Here's the drawing with two shaded views (mm, measured from the low corner). I have some questions. A direction names the side the tool comes from. Round coordinates to 2 decimals unless told otherwise and drop trailing zeros. Order: outer loops, then holes, each group sorted by start corner. A loop starts at its lowest first (then second) coordinate and runs counter-clockwise, first axis right, second up. Notation, with made-up numbers: (-24.5, -10) - (3.5, -10) arc R18 cw to (3.5, 6) - close; hole circle Ø7 at (0, 66). An arc over 180 degrees is marked (long way). One line per item, written item: value.
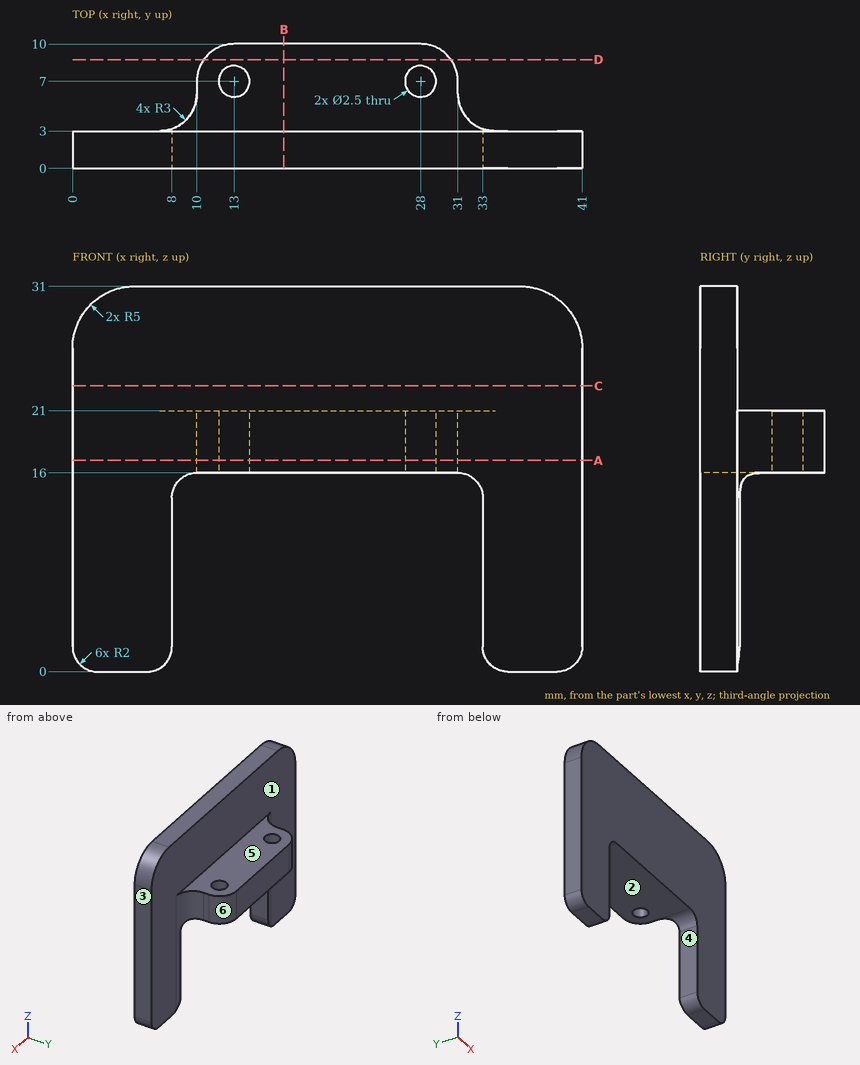
Q1. If we section it at C-C, the plane z = 23: Please give me the cut outline in (x, y), then the cut area to 3 significant figures.
Results list:
outline: (0, 0) - (41, 0) - (41, 3) - (0, 3) - close
area: 123 mm²
Q2. Will these pins go through, and if not, where does the flat tip stop? pin 1 (5.5 mm diameter, centred on x = 26.5, y = 5.5, fed in from +Z); pin 2 (1 mm diameter, centred on x = 29, z = 27.5, fed in from +Y); pin 3 (3 mm diameter, centred on x = 18.5, y = 6.5, fed in from -Z); pin 4 (0.8 mm diameter, centred on y = 6.5, z = 19, fed in from -X).
Results list:
pin 1: z = 31
pin 2: y = 3
pin 3: z = 16
pin 4: x = 10
Q3. If we section it at A-A, the plane z = 17: Please give me the cut outline in (x, y), then the cut area to 3 significant figures.
Results list:
outline: (0, 0) - (41, 0) - (41, 3) - (34, 3) arc R3 cw to (31, 6) - (31, 7) arc R3 ccw to (28, 10) - (13, 10) arc R3 ccw to (10, 7) - (10, 6) arc R3 cw to (7, 3) - (0, 3) - close; hole circle Ø2.5 at (13, 7); hole circle Ø2.5 at (28, 7)
area: 260 mm²
Q4. We'd pull the mould along X, two halves only. Please class the marked faces 4, 5 and 6: released by +X, released by -X, zero draft, split by the parting line, or undercut.
Results list:
face 4: undercut
face 5: zero draft
face 6: released by +X
Q5. If we section it at D-D, the plane y = 8.75: Please give me the cut outline in (x, z), then the cut area to 3 significant figures.
Results list:
outline: (10.56, 16) - (30.44, 16) - (30.44, 21) - (10.56, 21) - close
area: 99.4 mm²
Q6. If I drill on line 1 along Y through (x, z) = (13, 19.75); line 2 along X through (y, z) = (2, 2.5); line 3 along Y through (x, z) = (35, 3), over which ranges is the centre line in solid material (lowest first)?
Results list:
line 1: 0 to 5.75, 8.25 to 10
line 2: 0 to 8, 33 to 41
line 3: 0 to 3
Q7. Which directions (+Z, -Z, +X, -X, +Y, -Y) give clear straight access to the entire face, cutting with the end or side of a thin tool? Please do the marked faces 1, 2 and 3.
Results list:
face 1: +Z, +Y
face 2: -Z, +Y, -Y
face 3: +Z, -Z, +X, +Y, -Y
Q8. If we section it at B-B, the plane x = 17: Please give me the cut outline in (y, z).
Results list:
outline: (0, 16) - (10, 16) - (10, 21) - (3, 21) - (3, 31) - (0, 31) - close
